Part model, mm, in its own coordinate system. A direction names the side the tool comes from. Round coordinates to 2 decimals unless told otherwise and drop trailing zeros. Write each loop counter-clockwise with the first axis right and the second up, starting at its lowest first coordinate (ties: lowest second). Pieces come first, ordered by that corner, then holes. Notation, with made-up numbers: (22, -17) -> (57, -17) arc R35 cw to (57, 22) -> close; hole circle Ø8 at (-0.5, 65.25). An arc over 180 degrees is marked (long way). Return JSON: item names as keys, results as strings. Group by question number.
(1) Tool access for faces 1 (the cylindrical face through (2.326, -0.953, 4.93)), 2 (the flat face through (0, 1.2, 3)), 3 (the flat face through (0.1, 2.7, 3.5)): list every direction of +Z, -Z, +X, -X, +Y, -Y with a clear straight run to the whole face (end or side of a thin tool).
(2) Saw through at A-A (x = -3.4). List the corners of the cut face in (y, z) (3 decimals).
(3) Saw through at D-D (x = 1.75). List the corners of the cut face in (y, z).
(4) Drill centre lines: L1, parallel to Y at x = -2.5, z = 5; L2, parallel to X at y = -0.75, z = 2.75; L3, parallel to X at y = -1.75, z = 3. Where is each one in solid material? Low to high. Write a range as from..to.
(5) Saw through at C-C (y = -1). List the corners of the cut face in (x, z) (3 decimals), plus the area to 3 significant figures.
(6) Saw through at B-B (z = 4.75). List the corners of the cut face in (x, y) (3 decimals).
(7) Mould opens along Z. For faces 4 (the flat face through (0, 1, 10)), 5 (the flat face through (0, 2, 7)), 6 (the flat face through (-6.4, 1, 5)) say: +Z half, -Z half, draft (parallel to the pull), parting line (faces both ways), or undercut.
from build123d import *

# Parameters (mm, degrees)
BOSS_EXTRUDE1_DEPTH = 10
SKETCH1_3_W         = 12.8
SKETCH1_3_H         = 1.3
BOSS_EXTRUDE2_DEPTH = 7
SKETCH1_5_W         = 12.8
SKETCH1_5_H         = 1.3
CUT_EXTRUDE1_DEPTH  = 7
SKETCH1_6_R         = 1.075
CUT_EXTRUDE2_DEPTH  = 10
SKETCH4_W           = 12.8
SKETCH4_H           = 10
BOSS_EXTRUDE3_DEPTH = 1
CUT_EXTRUDE3_DEPTH  = 15
SKETCH8_W           = 12.8
SKETCH8_H           = 10
BOSS_EXTRUDE4_DEPTH = 1


with BuildPart() as part:
    # Sketch1 → Boss-Extrude1 (new body)
    with BuildSketch(Plane.XY):
        Polygon((6.4, 4), (-6.4, 4), (-6.4, -1), (-6.4, -4), (6.4, -4), (6.4, -1), align=None)
    extrude(amount=BOSS_EXTRUDE1_DEPTH)

    # Sketch1<3> → Boss-Extrude2 (add)
    with BuildSketch(Plane.XY):
        with Locations((0, 1.85)):
            Rectangle(SKETCH1_3_W, SKETCH1_3_H)
    extrude(amount=BOSS_EXTRUDE2_DEPTH)

    # Sketch1<5> → Cut-Extrude1 (cut)
    with BuildSketch(Plane.XY):
        with Locations((0, 1.85)):
            Rectangle(SKETCH1_5_W, SKETCH1_5_H)
    extrude(amount=CUT_EXTRUDE1_DEPTH, mode=Mode.SUBTRACT)

    # Sketch1<6> → Cut-Extrude2 (cut)
    with BuildSketch(Plane.XY):
        with Locations((3.4, -1)):
            Circle(SKETCH1_6_R)
        with Locations((-3.4, -1)):
            Circle(SKETCH1_6_R)
    extrude(amount=CUT_EXTRUDE2_DEPTH, mode=Mode.SUBTRACT)

    # Sketch4 → Boss-Extrude3 (add)
    with BuildSketch(Plane(origin=(0, 4, 0), x_dir=(1, 0, 0), z_dir=(0, 1, 0))):
        with Locations((0, -5)):
            Rectangle(SKETCH4_W, SKETCH4_H)
    extrude(amount=BOSS_EXTRUDE3_DEPTH)

    # Sketch6 → Cut-Extrude3 (cut)
    with BuildSketch(Plane(origin=(6.4, 0, 0), x_dir=(0, 0, -1), z_dir=(1, 0, 0))):
        Polygon((0, 2.5), (-7, 2.902751688), (-7, 2.5), align=None)
    extrude(amount=-CUT_EXTRUDE3_DEPTH, mode=Mode.SUBTRACT)

    # Sketch8 → Boss-Extrude4 (add)
    with BuildSketch(Plane(origin=(0, 5, 0), x_dir=(1, 0, 0), z_dir=(0, 1, 0))):
        with Locations((0, -5)):
            Rectangle(SKETCH8_W, SKETCH8_H)
    extrude(amount=BOSS_EXTRUDE4_DEPTH)


solid = part.part
Computed values:
{
 "1": {"face 1": "+Z, -Z", "face 2": "-Z, +X, -X", "face 3": "+X, -X"},
 "2": {"outline": "(-4, 0) -> (-2.075, 0) -> (-2.075, 10) -> (-4, 10) -> close; (0.075, 0) -> (1.2, 0) -> (1.2, 7) -> (2.903, 7) -> (2.5, 0) -> (6, 0) -> (6, 10) -> (0.075, 10) -> close"},
 "3": {"outline": "(-4, 0) -> (1.2, 0) -> (1.2, 7) -> (2.9, 7) -> (2.5, 0) -> (6, 0) -> (6, 10) -> (-4, 10) -> close"},
 "4": {"L1": "-4..-1.59, -0.41..1.2, 2.79..6", "L2": "-6.4..-4.45, -2.35..2.35, 4.45..6.4", "L3": "-6.4..-4.17, -2.63..2.63, 4.17..6.4"},
 "5": {"outline": "(-6.4, 0) -> (-4.475, 0) -> (-4.475, 10) -> (-6.4, 10) -> close; (-2.325, 0) -> (2.325, 0) -> (2.325, 10) -> (-2.325, 10) -> close; (4.475, 0) -> (6.4, 0) -> (6.4, 10) -> (4.475, 10) -> close", "area": "85.0 mm2"},
 "6": {"outline": "(-6.4, -4) -> (6.4, -4) -> (6.4, 1.2) -> (-6.4, 1.2) -> close; (-6.4, 2.773) -> (6.4, 2.773) -> (6.4, 6) -> (-6.4, 6) -> close; hole circle Ø2.15 at (-3.4, -1); hole circle Ø2.15 at (3.4, -1)"},
 "7": {"face 4": "+Z half", "face 5": "undercut", "face 6": "draft"}
}
